from build123d import *

# Parameters (mm, degrees)
DODANIE_WYCI_GNI_CIE1_START = 8
SZKIC2_R                    = 5
DODANIE_WYCI_GNI_CIE1_DEPTH = 10


with BuildPart() as part:
    # Szkic1 → Obrót1 (revolve)
    with BuildSketch(Plane.XY, mode=Mode.PRIVATE) as obr_t1_sk:
        Polygon((5, 0), (5, 2), (8.32, 2), (10.9, 0), align=None)
    revolve(obr_t1_sk.sketch.rotate(Axis((0, 0, 0), (0, 1, 0)), 90), axis=Axis((0, 0, 0), (0, 1, 0)))

    # Szkic2 → Dodanie-wyciągnięcie1 (add)
    with BuildSketch(Plane(origin=(0, 2, 0), x_dir=(1, 0, 0), z_dir=(0, 1, 0)).offset(DODANIE_WYCI_GNI_CIE1_START)):
        Polygon((0, 8.660254038), (-7.5, 4.330127019), (-7.5, -4.330127019), (0, -8.660254038), (7.5, -4.330127019), (7.5, 4.330127019), align=None)
        with Locations(Location((0, 0, 0), (0, 0, 90))):
            Circle(SZKIC2_R, mode=Mode.SUBTRACT)
    extrude(amount=-DODANIE_WYCI_GNI_CIE1_DEPTH)


solid = part.part
Can you work these out from the model? Positions are in its coordinate system, mm. A direction names the side the tool comes from. Give positions to 0.01 mm unless a question says otherwise; leave off trailing zeros. Loops run counter-clockwise (first coordinate to the right, second up) from the corner with the lowest first, then second, coordinate; pieces in that order, holes last. Notation, with made-up numbers: (-31.75, 28) - (5.25, 28) arc R14 cw to (5.25, 32) - close; hole circle Ø7 at (29.25, 0.5). An arc over 180 degrees is marked (long way). Answer as a JSON object with one key per item and string values.
Q1. Which directions (+Z, -Z, +X, -X, +Y, -Y) give clear straight access to the entire face, cutting with the end or side of a thin tool? Please do faces 1 (the flat face through (4, 2, -7)), 2 (the flat face through (4, 2, 7)), 3 (the flat face through (-4, 2, 7)), 4 (the flat face through (-3.698, 5.926, -6.526)).
Geometry says:
{"face 1": "-Z, +X, +Y", "face 2": "+Z, +X, +Y", "face 3": "+Z, -X, +Y", "face 4": "-Z, -X, +Y"}
Q2. Imagine slicing it at A-A on z = 0. Write out the boundary of the cut face in (x, y).
Geometry says:
{"outline": "(-10.9, 0) - (-5, 0) - (-5, 10) - (-7.5, 10) - (-7.5, 2) - (-8.32, 2) - close; (5, 0) - (10.9, 0) - (8.32, 2) - (7.5, 2) - (7.5, 10) - (5, 10) - close"}
Q3. Will these pins go through, and if not, where does the flat tip stop? P1, Ø0.7, axis at x = -8, z = -1.5, coming from the +Y side; P2, Ø2, axis at y = 2, z = -6.5, coming from the -X side; P3, Ø3, axis at y = 5.5, z = 7.5, coming from the +X side; P4, Ø2, axis at x = -3.5, z = -1, coming from the -Y side.
Geometry says:
{"P1": "y = 2", "P2": "x = -7.29", "P3": "x = 4.61", "P4": "through"}
Q4. Imagine slicing it at B-B on y = 7.5. Write out the boundary of the cut face in (x, z).
Geometry says:
{"outline": "(-7.5, -4.33) - (0, -8.66) - (7.5, -4.33) - (7.5, 4.33) - (0, 8.66) - (-7.5, 4.33) - close; hole circle Ø10 at (0, 0)"}
Q5. If I drill on L1, parallel to X at y = 5, z = 0; L2, parallel to Z at x = -3.25, y = 5; L3, parallel to Y at x = 8, z = -2.25, over which ranges is the centre line in solid material (lowest first)?
Geometry says:
{"L1": "-7.5 to -5, 5 to 7.5", "L2": "-6.78 to -3.8, 3.8 to 6.78", "L3": "0 to 2"}
Q6. If we mould it in two halves opening along Z, with no side actions, what happens to faces 5 (the cylindrical face through (4.88, 5.07, 1.08)), 6 (the flat face through (5, 0, -2)), 7 (the conical face through (3.248, 1.875, -7.835))? For each: pulls with the +Z half, pulls with the -Z half, needs draft (parallel to the pull), parting line crosses it, or undercut.
Geometry says:
{"face 5": "undercut", "face 6": "needs draft", "face 7": "parting line crosses it"}
